The drawing under review shows one solid part. Ordinate dimensions are in mm from its lowest x, y, z. A direction names the side the tool comes from. Coordinates: 2 decimals unless noted, no trailing zeros. Loops run counter-clockwise (first coordinate to the right, second up) from the corner with the lowest first, then second, coordinate; pieces in that order, holes last. Notation, with made-up numbers: (69.25, -23) - (110.25, -23) arc R29 ccw to (110.25, 16) - close; hole circle Ø10 at (-36.75, 53.25). An arc over 180 degrees is marked (long way). Use one line per item in the form item = value. Start each with the question number.
1. Add section D-D on z = 2.5. Give the boundary of the cut face in (x, y), and give its area (3 significant figures).
2. Add section C-C on z = 6.75. Give the boundary of the cut face in (x, y), and give its area (3 significant figures).
3. To check wall thickness, follow probe 1 along Y at (x, z) = (2.75, 7.15); probe 2 along Z at (x, y) = (1.3, 0.75); probe 3 along Z at (x, y) = (2.05, 3). State the ranges of each line that lie inside material, in increasing order.
4. For pin 1 Ø1 at (x, y) = (3, 2.5) entering from +Z; pin 2 Ø1.6 at (x, y) = (2.75, 2.75) entering from -Z; pin 3 Ø1.5 at (y, z) = (4.5, 5) entering from +X; pin 4 Ø3 at (y, z) = (3.5, 4) entering from +X, all flat-tipped, find the tip position at first contact; note any pin that passes through.
5. Draft analysis for pull direction Y (two halves, no side actions). For the marked faces 3, 4 and 5, state which applies: +Y half, -Y half, draft (parallel to the pull), parting line (faces both ways), or undercut.
6. Machinability: for the marked faces 1 and 2, which of the approach directions +Z, -Z, +X, -X, +Y, -Y give a long, thin tool a straight path to every point of the face, cutting with its end or side? Answer none if there is none.
7. Add section A-A on y = 2.75. Give the boundary of the cut face in (x, z), and give its area (3 significant figures).
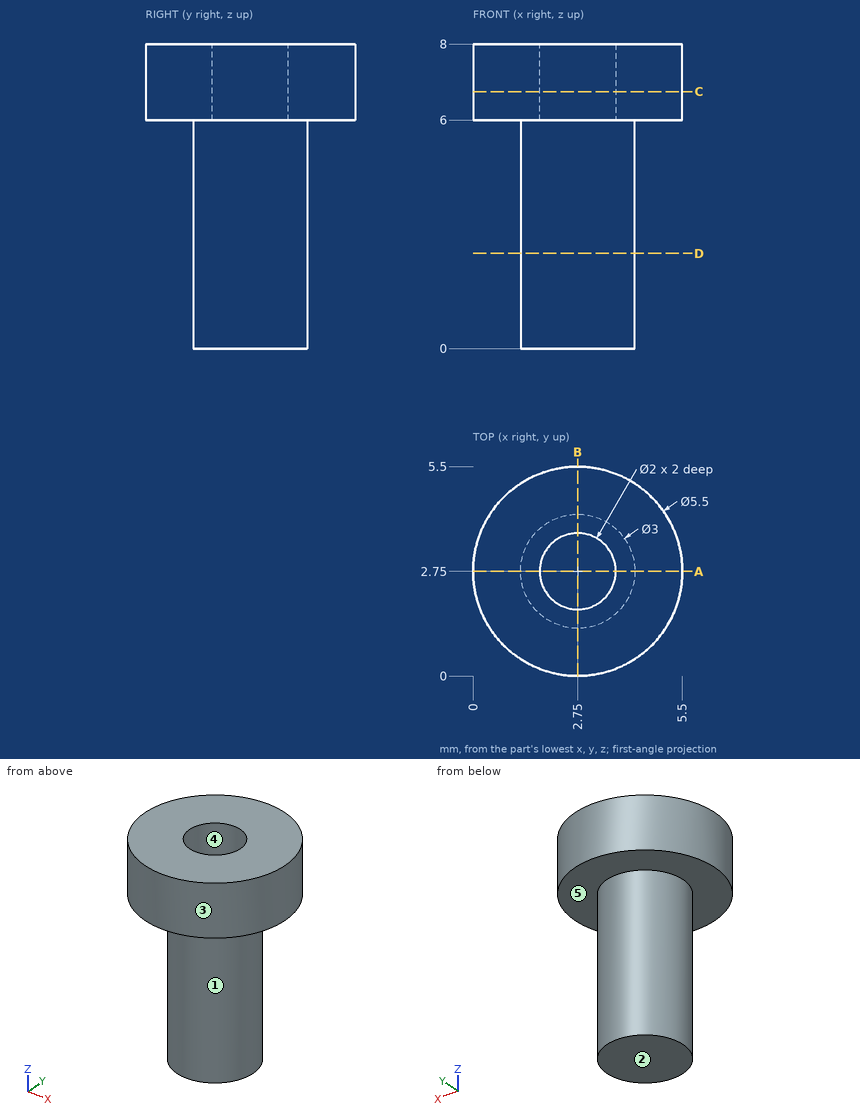
Conclusion:
q1.outline = circle Ø3 at (2.75, 2.75)
q1.area = 7.07 mm^2
q2.outline = circle Ø5.5 at (2.75, 2.75); hole circle Ø2 at (2.75, 2.75)
q2.area = 20.6 mm^2
q3.probe_1 = 0 to 1.75, 3.75 to 5.5
q3.probe_2 = 6 to 8
q3.probe_3 = 0 to 6
q4.pin_1 = 6
q4.pin_2 = 0
q4.pin_3 = 3.87
q4.pin_4 = 4.25
q5.face_3 = parting line
q5.face_4 = undercut
q5.face_5 = draft
q6.face_1 = -Z
q6.face_2 = -Z, +X, -X, +Y, -Y
q7.outline = (0, 6) - (1.25, 6) - (1.25, 0) - (4.25, 0) - (4.25, 6) - (5.5, 6) - (5.5, 8) - (3.75, 8) - (3.75, 6) - (1.75, 6) - (1.75, 8) - (0, 8) - close
q7.area = 25.0 mm^2
